Study the drawing (mm; zero at the part's minimum x, y, z) and answer. Give positions to 0.01 mm unless a question says otherwise; leave off trailing zeros. Loops run counter-clockwise (first coordinate to the right, second up) from the corner with the lowest first, then second, coordinate; pieces in that order, holes last. Notation, with made-up numbers: M 75.25,58 L 100.25,58 A30 ccw 100.25,84 Z; hole C 79,80.25 d10. An arc over 180 degrees is marked long. Return JSON: item names as keys, results as strings.
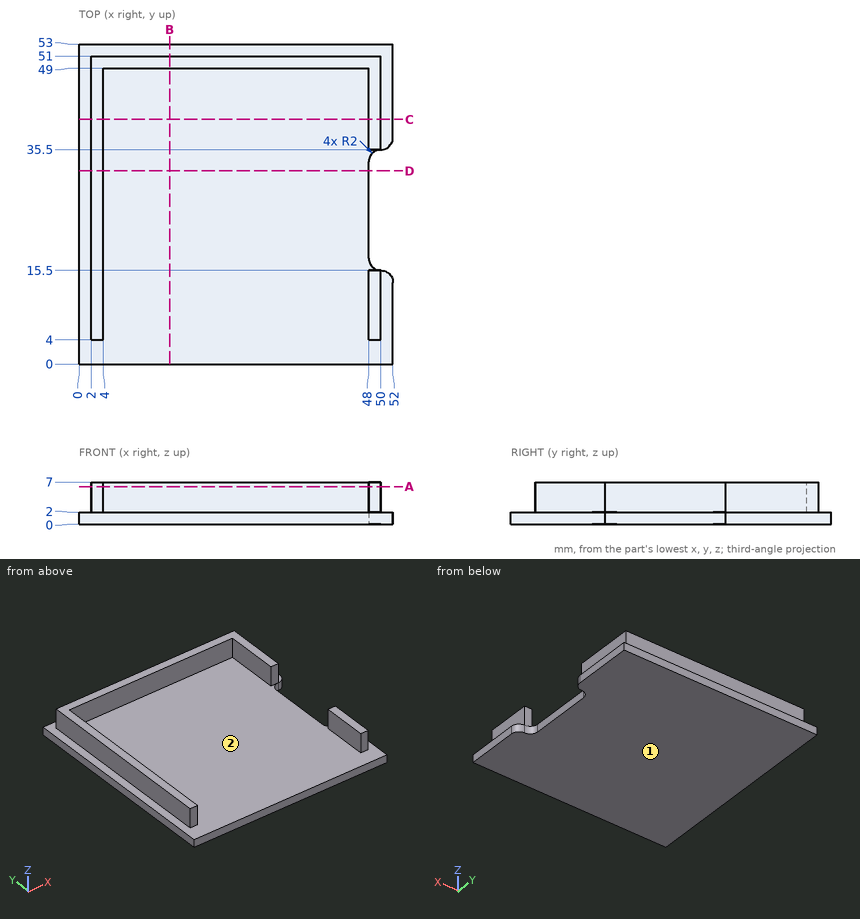
(1) Given pin 1 (4 mm diameter, centred on y = 32, z = 5.5, fed in from -X); pin 2 (2.5 mm diameter, centred on y = 40, z = 5.5, fed in from +X); pin 3 (2 mm diameter, centred on x = 48.5, z = 4.5, fed in from +Y), each flat-ended and moving along its own axis, determine where each tip first touches the part or whether it passes through.
Values follow:
{"pin 1": "x = 2", "pin 2": "x = 50", "pin 3": "y = 51"}
(2) Straight lines are drawn through the part: line 1 along X through (y, z) = (9, 5); line 2 along Z through (x, y) = (4.5, 18.5); line 3 along Y through (x, z) = (18, 4). For each, find the intervals that lie inside material, in ascending order.
Values follow:
{"line 1": "2 to 4, 48 to 50", "line 2": "0 to 2", "line 3": "49 to 51"}
(3) Determine the mould class of the marked faces 1 and 2 for opening direction X: released by +X, released by -X, zero draft, split by the parting line, or undercut.
Values follow:
{"face 1": "zero draft", "face 2": "undercut"}
(4) The part is cut by section D-D (y = 32). Determine the outline of the cut face in (x, z), and give its area (3 significant figures).
Values follow:
{"outline": "M 0,0 L 48,0 L 48,2 L 4,2 L 4,7 L 2,7 L 2,2 L 0,2 Z", "area": "106 mm²"}
(5) The part is cut by section C-C (y = 40.5). Determine the outline of the cut face in (x, z), and give its area (3 significant figures).
Values follow:
{"outline": "M 0,0 L 52,0 L 52,2 L 50,2 L 50,7 L 48,7 L 48,2 L 4,2 L 4,7 L 2,7 L 2,2 L 0,2 Z", "area": "124 mm²"}
(6) The part is cut by section A-A (z = 6.25). Determine the outline of the cut face in (x, y), and give its area (3 significant figures).
Values follow:
{"outline": "M 2,4 L 4,4 L 4,49 L 48,49 L 48,35.5 L 50,35.5 L 50,51 L 2,51 Z; M 48,4 L 50,4 L 50,15.5 L 48,15.5 Z", "area": "236 mm²"}
(7) The part is cut by section B-B (x = 15). Determine the outline of the cut face in (y, z), and give its area (3 significant figures).
Values follow:
{"outline": "M 0,0 L 53,0 L 53,2 L 51,2 L 51,7 L 49,7 L 49,2 L 0,2 Z", "area": "116 mm²"}
